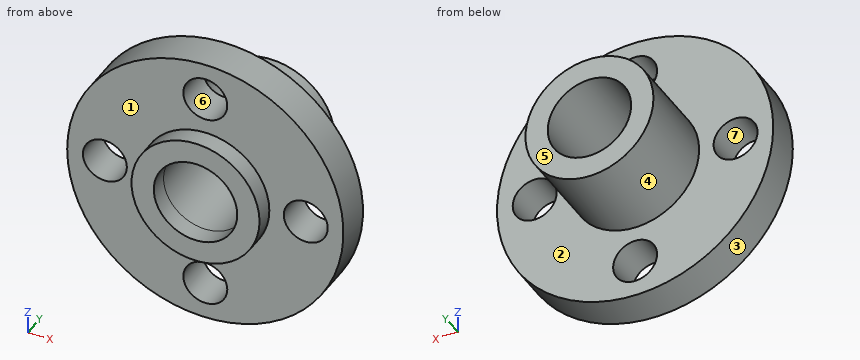
Autodesk Inventor part; units mm, degrees
ref_plane "YZ Plane" through (0, 0, 0) normal (1, 0, 0) x (0, 1, 0)
ref_plane "XZ Plane" through (0, 0, 0) normal (0, 1, 0) x (-1, 0, 0)
ref_plane "XY Plane" through (0, 0, 0) normal (0, 0, 1) x (1, 0, 0)
sketch "Sketch1" plane through (0, 0, 0) normal (0, 1, 0) x (-1, 0, 0)
  circle A0 centre (0, 0) radius 11
  circle A1 centre (0, 0) radius 5.1
  dimension "d0" = 22
  dimension "d1" = 10.2
extrude "Extrusion1" add sketch "Sketch1" along normal blind 3
extrude "Extrusion2" add sketch "Sketch1" along normal blind 10 contours A1
sketch "Sketch2" plane through (0, 10, 0) normal (0, 1, 0) x (1, 0, 0)
  circle A0 centre (0, 0) radius 5.1
hole "Hole1" at (0, 10, 0) direction (0, -1, 0) diameter 6.647 end through all
sketch "Sketch3" plane through (0, 0, 0) normal (0, -1, 0) x (1, 0, 0)
  circle A0 centre (0, 0) radius 5.1
  circle A1 centre (0, 0) radius 3.3235
  dimension "d13" = 10.2
extrude "Extrusion3" add sketch "Sketch3" along normal blind 1.5
sketch "Sketch4" plane through (0, 3, 0) normal (0, 1, 0) x (1, 0, 0)
  point P0 (0, 0)
  point P1 (8, 0)
  dimension "d16" = 8
hole "Hole2" at (8, 3, 0) direction (0, -1, 0) diameter 3.5 end through all
pattern_circular "Circular Pattern1" count 4 over 360 about axis through (0, -22.6803, 0) along (0, 1, 0) of "Hole2"
properties part number "DAI_OC"
Work out the finished part from the listing and answer in its coordinate system (mm). Face numbers are marked on the shaded views. A direction names the side the tool comes from. Coordinates: 2 decimals unless noted, no trailing zeros. Write each loop counter-clockwise with the first axis right and the second up, starting at its lowest first coordinate (ties: lowest second). Pieces come first, ordered by that corner, then holes.
Q1. A cutting plane is placed at A-A, the plane x = 0. Give the vertices of the cut face in (y, z).
Q2. Each of these flat-tipped pins is pushed along its axis until it touches: pin 1 Ø2 at (x, z) = (7, -4.5) entering from +Y; pin 2 Ø4 at (x, z) = (0, -8) entering from -Y; pin 3 Ø4 at (y, z) = (2.5, 4) entering from +X. Where does it stop, or does it pass through?
Q3. A cutting plane is placed at B-B, the plane z = 0. Give the vertices of the cut face in (x, y), then the cut area to 3 significant figures.
Q4. A cutting plane is placed at D-D, the plane z = 8. Give the vertices of the cut face in (x, y).
Q5. Which of the six approach directions +Z, -Z, +X, -X, +Y, -Y give full straight-line access (tool end or side, diameter ignored) to the marked faces 1, 2 and 3?
Q6. Find the intervals of material crossed by line 1 (Y direction, x = 1.5, z = -5); line 2 (Z direction, x = 2.5, y = 3.5); line 3 (Z direction, x = 3, y = 1.5), in increasing order.
Q7. A cutting plane is placed at C-C, the plane y = 5.25. Give the vertices of the cut face in (x, z).
Q8. Determine the mould class of the marked faces 4, 5, 6 and 7 for opening direction X: released by +X, released by -X, zero draft, split by the parting line, or undercut.
Findings below:
1. outline: (-1.5, -5.1) - (0, -5.1) - (0, -6.25) - (3, -6.25) - (3, -5.1) - (10, -5.1) - (10, -3.32) - (-1.5, -3.32) - close; (-1.5, 3.32) - (10, 3.32) - (10, 5.1) - (3, 5.1) - (3, 6.25) - (0, 6.25) - (0, 5.1) - (-1.5, 5.1) - close; (0, -11) - (3, -11) - (3, -9.75) - (0, -9.75) - close; (0, 9.75) - (3, 9.75) - (3, 11) - (0, 11) - close
2. pin 1: stops at y = 3
2. pin 2: stops at y = 0
2. pin 3: stops at x = 10.82
3. outline: (-11, 0) - (-9.75, 0) - (-9.75, 3) - (-11, 3) - close; (-6.25, 0) - (-5.1, 0) - (-5.1, -1.5) - (-3.32, -1.5) - (-3.32, 10) - (-5.1, 10) - (-5.1, 3) - (-6.25, 3) - close; (3.32, -1.5) - (5.1, -1.5) - (5.1, 0) - (6.25, 0) - (6.25, 3) - (5.1, 3) - (5.1, 10) - (3.32, 10) - close; (9.75, 0) - (11, 0) - (11, 3) - (9.75, 3) - close
3. area: 55.3 mm2
4. outline: (-7.55, 0) - (-1.75, 0) - (-1.75, 3) - (-7.55, 3) - close; (1.75, 0) - (7.55, 0) - (7.55, 3) - (1.75, 3) - close
5. face 1: -Y
5. face 2: +Y
5. face 3: +Y, -Y
6. line 1: y = 0 to 3
6. line 2: z = -4.45 to -2.19, 2.19 to 4.45
6. line 3: z = -10.58 to -1.43, 1.43 to 10.58
7. outline: circle Ø10.2 at (0, 0); hole circle Ø6.65 at (0, 0)
8. face 4: split by the parting line
8. face 5: zero draft
8. face 6: undercut
8. face 7: undercut
